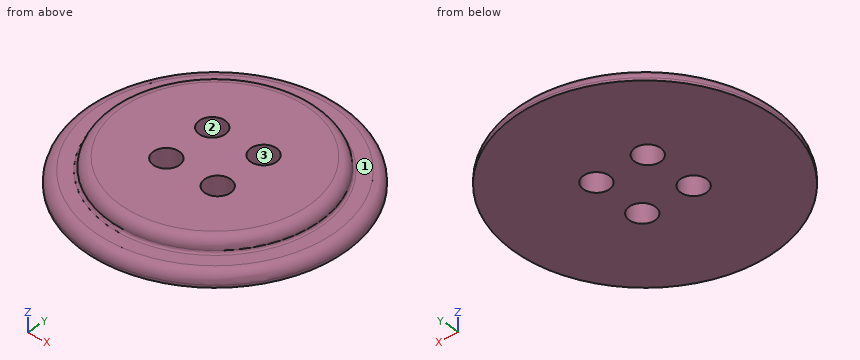
```python
from build123d import *

# Parameters (mm, degrees)
F2_R     = 25.4
F3_DEPTH = 50.8


with BuildPart() as f1:
    # F0 (on Front) → F1 (revolve)
    with BuildSketch(Plane.XZ):
        with BuildLine():
            Line((-254, 0), (0, 0))
            Line((0, 0), (0, 50.8))
            Line((0, 50.8), (-182.88, 50.8))
            ThreePointArc((-182.88, 50.8), (-197.24841, 44.84841), (-203.2, 30.48))
            ThreePointArc((-203.2, 30.48), (-204.687898, 26.887898), (-208.28, 25.4))
            Line((-208.28, 25.4), (-233.68, 25.4))
            ThreePointArc((-233.68, 25.4), (-248.04841, 19.44841), (-254, 5.08))
            Line((-254, 5.08), (-254, 0))
        make_face()
    revolve(axis=Axis((0, 0, 25.4), (0, 0, -1)))

    # F2 (on face) → F3 (cut)
    with BuildSketch(Plane.XY.offset(50.8)):
        with Locations((-50.8, 50.8)):
            Circle(F2_R)
        with Locations((50.8, 50.8)):
            Circle(F2_R)
        with Locations((-50.8, -50.8)):
            Circle(F2_R)
        with Locations((50.8, -50.8)):
            Circle(F2_R)
    extrude(amount=-F3_DEPTH, mode=Mode.SUBTRACT)


solid = f1.part
```
Design review of the part built by this model. Coordinates are the model's own, in mm. Face numbers are marked on the shaded views. Round coordinates to 2 decimals unless told otherwise and drop trailing zeros. Write each loop counter-clockwise with the first axis right and the second up, starting at its lowest first coordinate (ties: lowest second). Pieces come first, ordered by that corner, then holes.
Item 1: The part is to be moulded in two halves that separate along Y. For the marked faces 1, 2 and 3, say which applies: +Y half, -Y half, draft (parallel to the pull), parting line (faces both ways), or undercut.
Item 2: Clearance check with flat-ended pins moving along their axes: pin 1 Ø12 at (y, z) = (-38.5, 23.5) entering from +X; pin 2 Ø6 at (y, z) = (122.5, 22.5) entering from +X; pin 3 Ø4 at (x, z) = (9.5, 24.5) entering from -Y. State where each tip first meets the part, or that it passes through.
Item 3: We need section C-C on z = 15.5. Write out the cut boundary in (x, y).
Item 4: We need section A-A on y = 0. Write out the cut boundary in (x, z).
Item 5: For probe 1 along X at (y, z) = (72.5, 21.5); probe 2 along Y at (x, z) = (34.5, 39); probe 3 along Y at (x, z) = (-50.8, 16), list the stretches that pass through material, from the lowest coordinate up.
Returned:
1. face 1: draft
1. face 2: undercut
1. face 3: undercut
2. pin 1: stops at x = 246.87
2. pin 2: stops at x = 216.01
2. pin 3: stops at y = -243.96
3. outline: circle Ø502.25 at (0, 0); hole circle Ø50.8 at (-50.8, -50.8); hole circle Ø50.8 at (-50.8, 50.8); hole circle Ø50.8 at (50.8, -50.8); hole circle Ø50.8 at (50.8, 50.8)
4. outline: (-254, 0) - (254, 0) - (254, 5.08) arc R20.32 ccw to (233.68, 25.4) - (208.28, 25.4) arc R5.08 cw to (203.2, 30.48) arc R20.32 ccw to (182.88, 50.8) - (-182.88, 50.8) arc R20.32 ccw to (-203.2, 30.48) arc R5.08 cw to (-208.28, 25.4) - (-233.68, 25.4) arc R20.32 ccw to (-254, 5.08) - close
5. probe 1: x = -234.71 to -64, -37.6 to 37.6, 64 to 234.71
5. probe 2: y = -198.35 to -70.28, -31.32 to 31.32, 70.28 to 198.35
5. probe 3: y = -245.62 to -76.2, -25.4 to 25.4, 76.2 to 245.62
